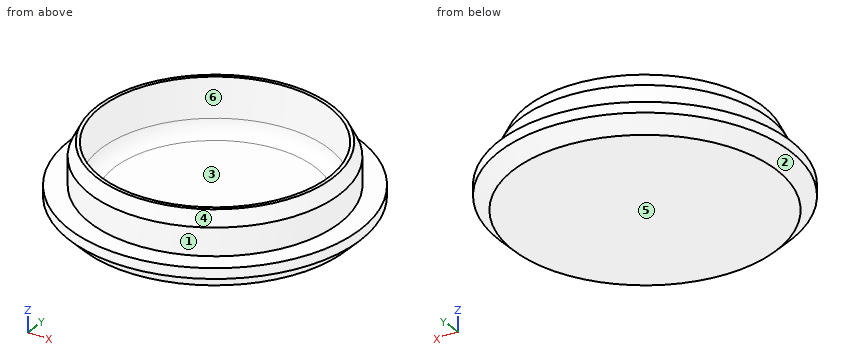
```python
from build123d import *

# Parameters (mm, degrees)
F2_R     = 2
F3_SIZE  = 2
F4_SIZE2 = 1
F4_SIZE  = 2


with BuildPart() as f1:
    # F0 (on Front) → F1 (revolve)
    with BuildSketch(Plane.XZ):
        Polygon((-18, 3.5), (-21, 3.5), (-21, 0), (0, 0), (0, 1.7), (-16.5, 1.7), (-16.5, 9.5), (-18, 9.5), align=None)
    revolve(axis=Axis((0, 0, 0.85), (0, 0, -1)))

    # F2
    f2_edges = [f1.edges().sort_by_distance(p)[0] for p in [
        (16.5, 0, 1.7),
    ]]
    fillet(f2_edges, radius=F2_R)

    # F3
    f3_edges = [f1.edges().sort_by_distance(p)[0] for p in [
        (21, 0, 0),
    ]]
    chamfer(f3_edges, length=F3_SIZE)

    # F4
    f4_edges = [f1.edges().sort_by_distance(p)[0] for p in [
        (18, 0, 9.5),
    ]]
    f4_side = f1.faces().sort_by_distance((18, 0, 6.5))[0]
    chamfer(f4_edges, length=F4_SIZE, length2=F4_SIZE2, reference=f4_side)


solid = f1.part
```
For this review, take the finished solid that the model builds, in its own axes (mm). Face numbers are marked on the shaded views. A direction names the side the tool comes from. Round coordinates to 2 decimals unless told otherwise and drop trailing zeros. Write each loop counter-clockwise with the first axis right and the second up, starting at its lowest first coordinate (ties: lowest second). Pieces come first, ordered by that corner, then holes. Notation, with made-up numbers: (48.25, -15.75) - (66.25, -15.75) arc R13 ccw to (66.25, -2.75) - close; hole circle Ø2 at (84.25, -7). An arc over 180 degrees is marked (long way). Write each question's results on one line, items separated by ' | '.
Item 1: Take a section at A-A on x = 0. State the section outline as (y, z) points.
Calculated:
outline: (-21, 2) - (-19, 0) - (19, 0) - (21, 2) - (21, 3.5) - (18, 3.5) - (18, 7.5) - (17, 9.5) - (16.5, 9.5) - (16.5, 3.7) arc R2 cw to (14.5, 1.7) - (-14.5, 1.7) arc R2 cw to (-16.5, 3.7) - (-16.5, 9.5) - (-17, 9.5) - (-18, 7.5) - (-18, 3.5) - (-21, 3.5) - close
Item 2: Draft analysis for pull direction X (two halves, no side actions). For the marked faces 3, 4, 5 and 6, state which applies: pulls with the +X half, pulls with the -X half, needs draft (parallel to the pull), parting line crosses it, or undercut.
Calculated:
face 3: undercut | face 4: parting line crosses it | face 5: needs draft | face 6: undercut
Item 3: Take a section at D-D on z = 4.5. State the section outline as (x, y) points, then the cut area to 3 significant figures.
Calculated:
outline: circle Ø36 at (0, 0); hole circle Ø33 at (0, 0) | area: 163 mm^2
Item 4: For the marked faces 1 and 2, list the 3-axis set-ups (+Z, -Z, +X, -X, +Y, -Y) from which the entire face can be reached by the end or side of a thin tool; tool diameter is ignored.
Calculated:
face 1: +Z | face 2: -Z
Item 5: To check wall thickness, follow line 1 along Y through (x, z) = (0, 6.1); line 2 along X through (y, z) = (14, 4.5); line 3 along Y through (x, z) = (11, 8). State the ranges of each line that lie inside material, in increasing order. Write a range as from..to.
Calculated:
line 1: y = -18..-16.5, 16.5..18 | line 2: x = -11.31..-8.73, 8.73..11.31 | line 3: y = -13.93..-12.3, 12.3..13.93
Item 6: Take a section at C-C on z = 8. State the section outline as (x, y) points.
Calculated:
outline: circle Ø35.5 at (0, 0); hole circle Ø33 at (0, 0)
Item 7: For pin 1 (2 mm diameter, centred on x = -9.5, z = 2, fed in from -Y); pin 2 (2 mm diameter, centred on x = 3.5, z = 6.5, fed in from -Y); pin 3 (1.5 mm diameter, centred on x = 16.5, y = -13, fed in from -Z), all flat-tipped, find the tip position at first contact; note any pin that passes through.
Calculated:
pin 1: stops at y = -19.2 | pin 2: stops at y = -17.83 | pin 3: stops at z = 1.26
